```python
from build123d import *

# Parameters (mm, degrees)
SZKIC1_W               = 20.5
SZKIC1_H               = 10
OTW_R_GWINTOWANY_M81_D = 6.8


with BuildPart() as part:
    # Szkic1 → Obrót1 (revolve)
    with BuildSketch(Plane.XY, mode=Mode.PRIVATE) as obr_t1_sk:
        with Locations((-52.25, -1.619007804)):
            Rectangle(SZKIC1_W, SZKIC1_H)
    revolve(obr_t1_sk.sketch.rotate(Axis((0, 12.15490524, 0), (0, -1, 0)), 270), axis=Axis((0, 12.15490524, 0), (0, -1, 0)))

    # Otwór gwintowany M81 (through all)
    with Locations(Plane(origin=(-20.058639265, 3.380992196, -48.425838957), x_dir=(0, 0, 1), z_dir=(0, 1, 0))):
        with Locations((0, 0), (0, 40.11727853), (28.367199692, 68.484478222), (68.484478222, 68.484478222), (96.851677914, 40.11727853), (96.851677914, 0), (68.484478222, -28.367199692), (28.367199692, -28.367199692)):
            Hole(OTW_R_GWINTOWANY_M81_D / 2)


solid = part.part
```
Input: part model. Units: mm. Frame: model coordinates. Coordinates: 2 decimals unless noted, no trailing zeros. Write each loop counter-clockwise with the first axis right and the second up, starting at its lowest first coordinate (ties: lowest second). Pieces come first, ordered by that corner, then holes. Notation, with made-up numbers: (71, 33) -> (108, 33) arc R22 cw to (108, 68) -> close; hole circle Ø9 at (14, -24). An arc over 180 degrees is marked (long way). Answer as a JSON object with one key per item and string values.
1. Mould query, pull axis X, two halves, no side actions, for faces 1 (the face through (13, 3.381, 41)), 2 (the face through (-12.62, -1.55, 40.06)), 3 (the face through (-2.75, -1.55, -62.44)). Classes: released by +X, released by -X, zero draft, split by the parting line, or undercut.
Result set:
{"face 1": "zero draft", "face 2": "undercut", "face 3": "split by the parting line"}
2. Section B-B on z = 0. Return the cut outline in (x, y).
Result set:
{"outline": "(-62.5, -6.62) -> (-42, -6.62) -> (-42, 3.38) -> (-62.5, 3.38) -> close; (42, -6.62) -> (62.5, -6.62) -> (62.5, 3.38) -> (42, 3.38) -> close"}
3. Section C-C on y = -1.25. Count the separate pieces of the cut face and the enclosed holes in it, then the cut area to 3 significant figures.
Result set:
{"separate pieces": "1", "enclosed holes": "9", "area": "6,440 mm2"}
4. Section D-D on x = 21.5. Return the cut outline in (y, z).
Result set:
{"outline": "(-6.62, -58.69) -> (3.38, -58.69) -> (3.38, -51.51) -> (-6.62, -51.51) -> close; (-6.62, -45.35) -> (3.38, -45.35) -> (3.38, -36.08) -> (-6.62, -36.08) -> close; (-6.62, 36.08) -> (3.38, 36.08) -> (3.38, 45.35) -> (-6.62, 45.35) -> close; (-6.62, 51.51) -> (3.38, 51.51) -> (3.38, 58.69) -> (-6.62, 58.69) -> close"}
5. Material intervals for line 1 (X direction, y = -0.5, z = -17.5); line 2 (Z direction, x = -22, y = 0.5); line 3 (Z direction, x = -50.5, y = -3), sorted ascending. Write a range as from..to.
Result set:
{"line 1": "x = -60..-50.66, -46.19..-38.18, 38.18..46.19, 50.66..60", "line 2": "z = -58.5..-51.22, -45.63..-35.78, 35.78..45.63, 51.22..58.5", "line 3": "z = -36.82..-22.75, -17.36..17.36, 22.75..36.82"}
6. Section A-A on x = 0. Return the cut outline in (y, z).
Result set:
{"outline": "(-6.62, -62.5) -> (3.38, -62.5) -> (3.38, -42) -> (-6.62, -42) -> close; (-6.62, 42) -> (3.38, 42) -> (3.38, 62.5) -> (-6.62, 62.5) -> close"}
7. First-contact query: P1, Ø1, axis at x = 21.5, y = -5, coming from the +Z side; P2, Ø9, axis at x = 20.06, z = -48.43, coming from the +Y side; P3, Ø5, axis at y = -3.5, z = -15.5, coming from the -X side; P4, Ø1, axis at x = -11.5, y = 0.5, coming from the -Z side. Flat tips, straight axial feed; report the tip coordinate or a pass-through.
Result set:
{"P1": "stops at z = 58.87", "P2": "stops at y = 3.38", "P3": "stops at x = -61.13", "P4": "stops at z = -61.52"}
